Job drawing, mm, ordinate dimensions from the low corner. One solid piece. Coordinates: 2 decimals unless noted, no trailing zeros. Write each loop counter-clockwise with the first axis right and the second up, starting at its lowest first coordinate (ties: lowest second). Pieces come first, ordered by that corner, then holes.
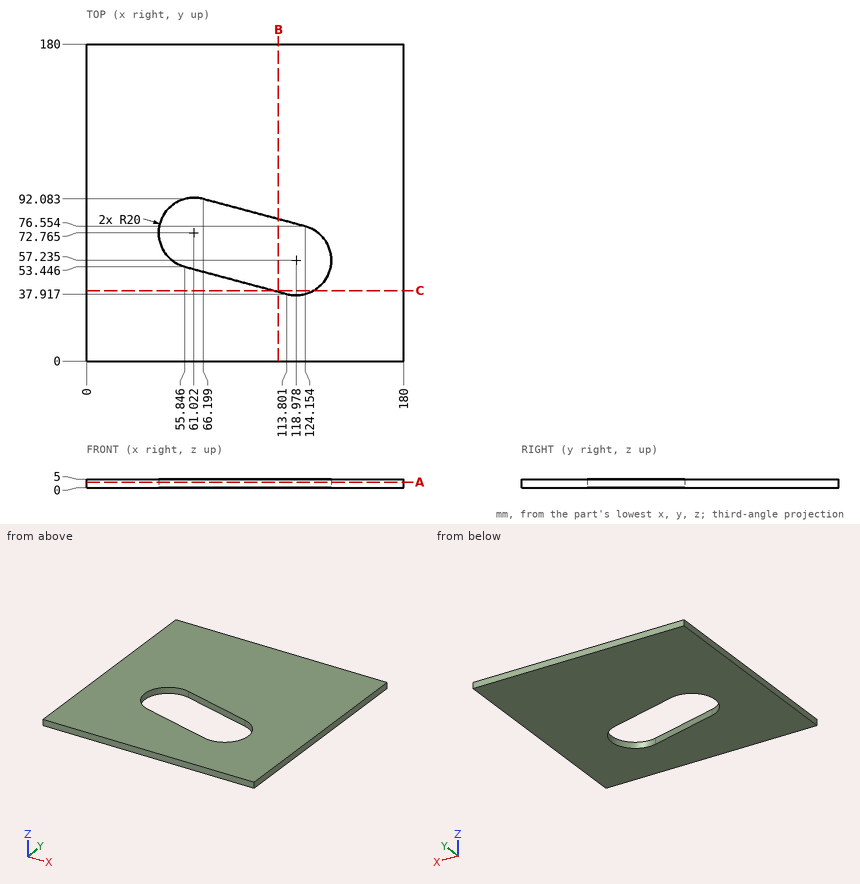
1. Probe line 1 along Y through (x, z) = (46, 1.15); line 2 along Y through (x, z) = (44.5, 4.5) (1 decimal); line 3 along X through (y, z) = (58.5, 3.3) (1 decimal). List the from-to ranges inside material, lowest first.
Computed values:
line 1: y = 0 to 59.56, 85.97 to 180
line 2: y = 0 to 61.5, 84 to 180
line 3: x = 0 to 47, 138.9 to 180
2. Saw through at C-C on y = 40. List the corners of the cut face in (x, z).
Computed values:
outline: (0, 0) - (106.03, 0) - (106.03, 5) - (0, 5) - close; (129.12, 0) - (180, 0) - (180, 5) - (129.12, 5) - close
3. Saw through at B-B on x = 109. List the corners of the cut face in (y, z) (1 decimal), plus the area to 3 significant figures.
Computed values:
outline: (0, 0) - (39.2, 0) - (39.2, 5) - (0, 5) - close; (80.6, 0) - (180, 0) - (180, 5) - (80.6, 5) - close
area: 693 mm2
4. Saw through at A-A on z = 3.2. List the corners of the cut face in (x, y) (1 decimal).
Computed values:
outline: (0, 0) - (180, 0) - (180, 180) - (0, 180) - close; hole (55.8, 53.4) - (113.8, 37.9) arc R20 ccw to (124.2, 76.6) - (66.2, 92.1) arc R20 ccw to start
